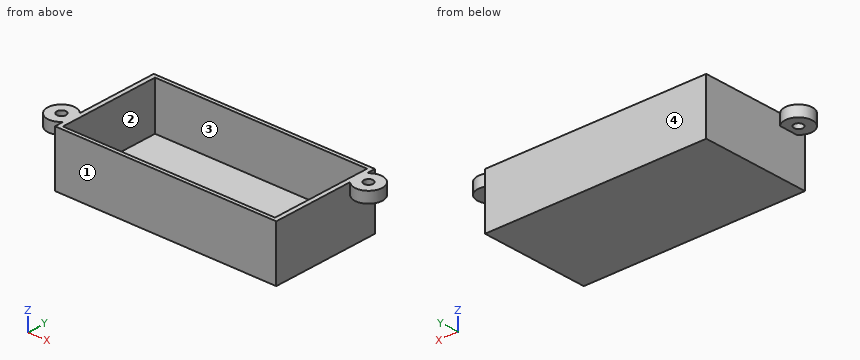
from build123d import *

# Parameters (mm, degrees)
SKIZZE1_W                       = 60.5
SKIZZE1_H                       = 30
AUFSATZ_LINEAR_AUSTRAGEN1_DEPTH = 15
SKIZZE2_W                       = 58
SKIZZE2_H                       = 28
SKIZZE2_R                       = 1.25
SCHNITT_LINEAR_AUSTRAGEN2_DEPTH = 13
SKIZZE2_5_R                     = 1.25
AUFSATZ_LINEAR_AUSTRAGEN2_DEPTH = 3


with BuildPart() as part:
    # Skizze1 → Aufsatz-Linear austragen1 (new body)
    with BuildSketch(Plane.XY):
        Rectangle(SKIZZE1_W, SKIZZE1_H)
    extrude(amount=AUFSATZ_LINEAR_AUSTRAGEN1_DEPTH)

    # Skizze2 → Schnitt-Linear austragen2 (cut)
    # profile 1 of 3: a face of its own
    with BuildSketch(Plane.XY.offset(15)):
        Rectangle(SKIZZE2_W, SKIZZE2_H)
    # profile 2 of 3: a face of its own
    with BuildSketch(Plane.XY.offset(15)):
        with BuildLine():
            Line((-30.25, -7.450490243), (-30.25, -12.549509757))
            ThreePointArc((-30.25, -12.549509757), (-36.75, -10), (-30.25, -7.450490243))
        make_face()
        with Locations((-33, -10)):
            Circle(SKIZZE2_R, mode=Mode.SUBTRACT)
    # profile 3 of 3: a face of its own
    with BuildSketch(Plane.XY.offset(15)):
        with BuildLine():
            Line((30.25, 12.549509757), (30.25, 7.450490243))
            ThreePointArc((30.25, 7.450490243), (36.75, 10), (30.25, 12.549509757))
        make_face()
        with Locations((33, 10)):
            Circle(SKIZZE2_R, mode=Mode.SUBTRACT)
    extrude(amount=-SCHNITT_LINEAR_AUSTRAGEN2_DEPTH, mode=Mode.SUBTRACT)

    # Skizze2<5> → Aufsatz-Linear austragen2 (add)
    # profile 1 of 2: a face of its own
    with BuildSketch(Plane.XY.offset(15)):
        with BuildLine():
            Line((-30.25, -12.549509757), (-30.25, -7.450490243))
            ThreePointArc((-30.25, -7.450490243), (-36.75, -10), (-30.25, -12.549509757))
        make_face()
        with Locations((-33, -10)):
            Circle(SKIZZE2_5_R, mode=Mode.SUBTRACT)
    # profile 2 of 2: a face of its own
    with BuildSketch(Plane.XY.offset(15)):
        with BuildLine():
            ThreePointArc((30.25, 7.450490243), (36.75, 10), (30.25, 12.549509757))
            Line((30.25, 12.549509757), (30.25, 7.450490243))
        make_face()
        with Locations((33, 10)):
            Circle(SKIZZE2_5_R, mode=Mode.SUBTRACT)
    extrude(amount=-AUFSATZ_LINEAR_AUSTRAGEN2_DEPTH)


solid = part.part
The listing builds one solid part. Answer for the finished solid, in the listing's coordinates (mm). Face numbers are marked on the shaded views. A direction names the side the tool comes from. Coordinates: 2 decimals unless noted, no trailing zeros. Loops run counter-clockwise (first coordinate to the right, second up) from the corner with the lowest first, then second, coordinate; pieces in that order, holes last. Notation, with made-up numbers: M 46,19.5 L 84,19.5 A23 ccw 84,39.5 Z; hole C 80,-19 d2. An arc over 180 degrees is marked long. Answer in a Markdown table with one row per item.
1) Find section C-C (y = 10). Determine the outline of the cut face in (x, z), then the cut area to 4 significant figures.
Answers below:
| item | result |
|---|---|
| outline | M -30.25,0 L 30.25,0 L 30.25,12 L 31.75,12 L 31.75,15 L 29,15 L 29,2 L -29,2 L -29,15 L -30.25,15 Z; M 34.25,12 L 36.75,12 L 36.75,15 L 34.25,15 Z |
| area | 165.5 mm^2 |
2) Find the intervals of material crossed by probe 1 along X at (y, z) = (-5.75, 10); probe 2 along Y at (x, z) = (0, 10.75); probe 3 along Y at (x, z) = (33, 12.95), in increasing order.
Answers below:
| item | result |
|---|---|
| probe 1 | -30.25 to -29, 29 to 30.25 |
| probe 2 | -15 to -14, 14 to 15 |
| probe 3 | 6.25 to 8.75, 11.25 to 13.75 |
3) Which of the six approach directions +Z, -Z, +X, -X, +Y, -Y give full straight-line access (tool end or side, diameter ignored) to the marked faces 1 and 2?
Answers below:
| item | result |
|---|---|
| face 1 | +Z, -Z, +X, -X, -Y |
| face 2 | +Z |
4) Find section D-D (x = -4). Determine the outline of the cut face in (y, z).
Answers below:
| item | result |
|---|---|
| outline | M -15,0 L 15,0 L 15,15 L 14,15 L 14,2 L -14,2 L -14,15 L -15,15 Z |
5) Determine the mould class of the marked faces 3 and 4 for opening direction X: released by +X, released by -X, zero draft, split by the parting line, or undercut.
Answers below:
| item | result |
|---|---|
| face 3 | undercut |
| face 4 | zero draft |
6) Given pin 1 (5 mm diameter, centred on x = -33.5, y = -10.5, fed in from -Z); pin 2 (6 mm diameter, centred on y = -3.5, z = 7.5, fed in from +X), each flat-ended and moving along its own axis, determine where each tip first touches the part or whether it passes through.
Answers below:
| item | result |
|---|---|
| pin 1 | z = 12 |
| pin 2 | x = 30.25 |
7) Find section A-A (x = -33). Determine the outline of the cut face in (y, z), then the cut area to 3 significant figures.
Answers below:
| item | result |
|---|---|
| outline | M -13.75,12 L -11.25,12 L -11.25,15 L -13.75,15 Z; M -8.75,12 L -6.25,12 L -6.25,15 L -8.75,15 Z |
| area | 15.0 mm^2 |
8) Find section B-B (z = 5). Determine the outline of the cut face in (x, y).
Answers below:
| item | result |
|---|---|
| outline | M -30.25,-15 L 30.25,-15 L 30.25,15 L -30.25,15 Z; hole M -29,-14 L 29,-14 L 29,14 L -29,14 Z |
